Could you check a few things on this model? Use its own coordinates, in mm. Round coordinates to 2 decimals unless told otherwise and drop trailing zeros. Loops run counter-clockwise (first coordinate to the right, second up) from the corner with the lowest first, then second, coordinate; pieces in that order, holes last.
from build123d import *

# Parameters (mm, degrees)
F1_DEPTH = 450
F2_W     = 12.7
F2_H     = 5
F3_DEPTH = 900
F4_R     = 2


with BuildPart() as f1:
    # F0 (on Right) → F1 (new body, symmetric)
    with BuildSketch(Plane.YZ):
        Polygon((20, 2.5), (20, 10), (12.5, 10), (12.5, 3.65), (7.5, 3.65), (7.5, 10), (-7.5, 10), (-7.5, 3.65), (-12.5, 3.65), (-12.5, 10), (-20, 10), (-20, 2.5), (-13.65, 2.5), (-13.65, -2.5), (-20, -2.5), (-20, -10), (-12.5, -10), (-12.5, -3.65), (-7.5, -3.65), (-7.5, -10), (7.5, -10), (7.5, -3.65), (12.5, -3.65), (12.5, -10), (20, -10), (20, -2.5), (13.65, -2.5), (13.65, 2.5), align=None)
    extrude(amount=F1_DEPTH, both=True)

    # F2 (on face) → F3 (cut)
    with BuildSketch(Plane(origin=(-450, 0, 0), x_dir=(0, -1, 0), z_dir=(-1, 0, 0))):
        Rectangle(F2_W, F2_H)
    extrude(amount=-F3_DEPTH, mode=Mode.SUBTRACT)

    # F4
    f4_edges = [f1.edges().sort_by_distance(p)[0] for p in [
        (0, 20, 10),
        (0, -20, -10),
        (0, 20, -10),
        (0, -20, 10),
    ]]
    fillet(f4_edges, radius=F4_R)


solid = f1.part
Item 1: If we section it at A-A, the plane y = 0: Please give me the cut outline in (x, z), then the cut area to 3 significant figures.
Results list:
outline: (-450, -10) - (450, -10) - (450, -2.5) - (-450, -2.5) - close; (-450, 2.5) - (450, 2.5) - (450, 10) - (-450, 10) - close
area: 13,500 mm2
Item 2: Will these pins go through, and if not, where does the flat tip stop? pin 1 (1.5 mm diameter, centred on x = 185, y = 9.5, fed in from +Z); pin 2 (2 mm diameter, centred on x = -160.5, z = 0, fed in from +Y); pin 3 (1.5 mm diameter, centred on x = 75, z = -1, fed in from -Y).
Results list:
pin 1: stops at z = 3.65
pin 2: stops at y = 13.65
pin 3: stops at y = -13.65
Item 3: If I drill on line 1 along Y through (x, z) = (162, -5.5); line 2 along Z through (x, y) = (278, -15); line 3 along Y through (x, z) = (62, 1.5), over which ranges is the centre line in solid material (lowest first)?
Results list:
line 1: y = -20 to -12.5, -7.5 to 7.5, 12.5 to 20
line 2: z = -10 to -2.5, 2.5 to 10
line 3: y = -13.65 to -6.35, 6.35 to 13.65
